The figure shows three views and two pictorial views of one solid part (mm, origin at its lowest corner). Answer the questions. A direction names the side the tool comes from. Coordinates: 2 decimals unless noted, no trailing zeros. Loops run counter-clockwise (first coordinate to the right, second up) from the corner with the lowest first, then second, coordinate; pieces in that order, holes last. Notation, with made-up numbers: M 53.25,42.25 L 71.25,42.25 A28 ccw 71.25,81.25 Z; hole C 88.5,65 d4. An arc over 180 degrees is marked long. Answer in a Markdown table with one row per item. Add a question column.
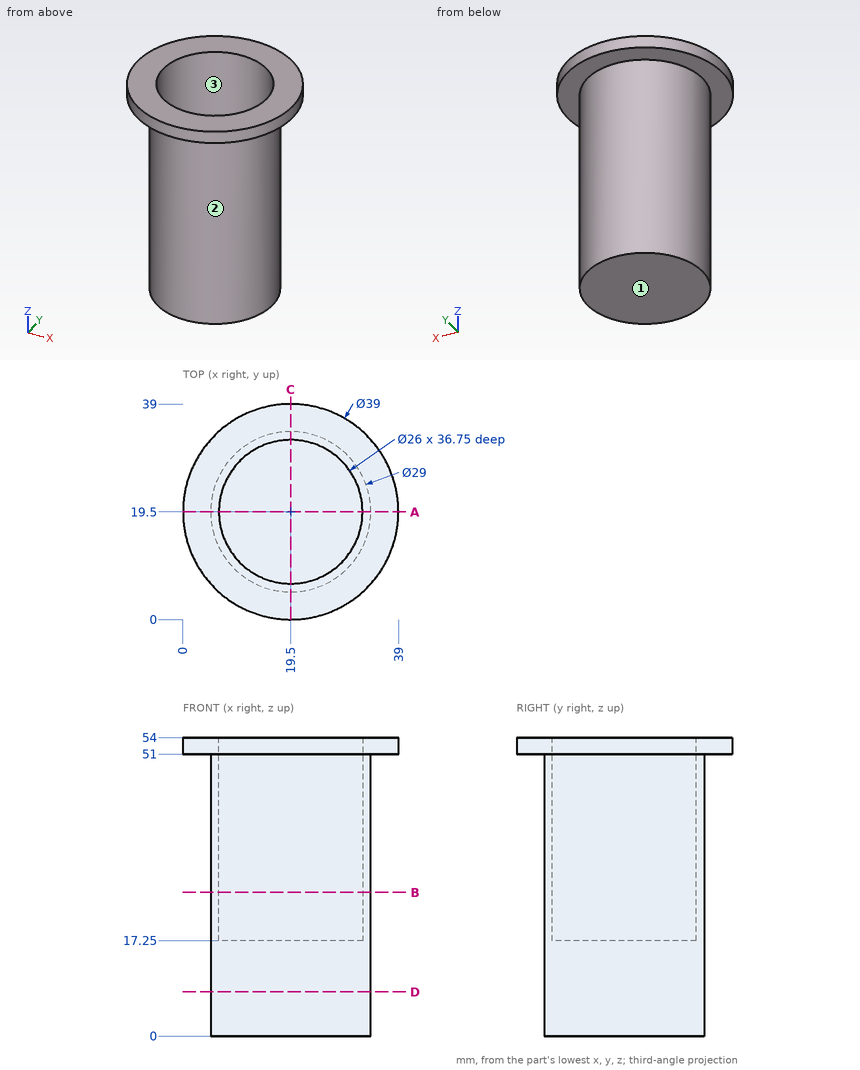
(1) A cutting plane is placed at D-D (z = 8). Give the vertices of the cut face in (x, y).
(2) Each of these flat-tipped pins is pushed along its axis until it touches: pin 1 (8 mm diameter, centred on x = 20.5, z = 43.5, fed in from +Y); pin 2 (2 mm diameter, centred on x = 6.5, y = 5, fed in from -Z); pin 3 (21 mm diameter, centred on x = 19.5, y = 19.5, fed in from +Z). Where does it stop, or does it pass through?
(3) Straight lines are drawn through the part: line 1 (Y direction, x = 19, z = 32); line 2 (X direction, y = 20, z = 51.5); line 3 (Z direction, x = 16.5, y = 20). For each, find the intervals that lie inside material, in ascending order.
(4) For the marked faces 1, 2 and 3, determine the directions among +Z, -Z, +X, -X, +Y, -Y from which every point of the face is accessible in a straight line to the end or side of a thin tool.
(5) A cutting plane is placed at B-B (z = 26). Give the vertices of the cut face in (x, y), plus the area to 3 significant figures.
(6) A cutting plane is placed at A-A (y = 19.5). Give the vertices of the cut face in (x, z), plus the area to 4 significant figures.
Solved:
| question | item | result |
|---|---|---|
| 1 | outline | C 19.5,19.5 d29 |
| 2 | pin 1 | stops at y = 34 |
| 2 | pin 2 | stops at z = 51 |
| 2 | pin 3 | stops at z = 17.25 |
| 3 | line 1 | y = 5.01 to 6.51, 32.49 to 33.99 |
| 3 | line 2 | x = 0.01 to 6.51, 32.49 to 38.99 |
| 3 | line 3 | z = 0 to 17.25 |
| 4 | face 1 | -Z, +X, -X, +Y, -Y |
| 4 | face 2 | -Z |
| 4 | face 3 | +Z |
| 5 | outline | C 19.5,19.5 d29; hole C 19.5,19.5 d26 |
| 5 | area | 130 mm² |
| 6 | outline | M 0,51 L 5,51 L 5,0 L 34,0 L 34,51 L 39,51 L 39,54 L 32.5,54 L 32.5,17.25 L 6.5,17.25 L 6.5,54 L 0,54 Z |
| 6 | area | 640.5 mm² |
